Work out the finished part from the listing and answer in its coordinate system (mm). A direction names the side the tool comes from. Coordinates: 2 decimals unless noted, no trailing zeros. Order: outer loops, then holes, each group sorted by start corner. A loop starts at its lowest first (then second) coordinate and runs counter-clockwise, first axis right, second up. Notation, with made-up numbers: (68, -16) -> (104, -16) arc R16 cw to (104, -9) -> close; hole circle Ø10 at (80.5, 12.25). An arc over 180 degrees is marked (long way). Answer as CSV lines item,"result". Start each with the question number.
Item 1: Which of the six approach directions +Z, -Z, +X, -X, +Y, -Y give full straight-line access (tool end or side, diameter ignored) to faces 1 (the face through (1.972, -8.5, -5.156)), 2 (the face through (1.972, 6.461, -7.513)), 3 (the face through (1.972, 9.907, -0.825))?
Item 2: Section C-C (x = 4.75) is taken. Write down the section's boundary in (y, z).
Item 3: Each of these flat-tipped pins is pushed along its axis until it touches: pin 1 Ø4 at (x, y) = (19.5, 3) entering from +Z; pin 2 Ø6 at (x, z) = (8.5, -7.5) entering from +Y; pin 3 Ø2 at (x, y) = (20.5, 0) entering from -Z. Where does it stop, or does it pass through?
Item 4: Straight lines are drawn through the part: L1, parallel to X at y = -1, z = 6.25; L2, parallel to Y at x = 22.25, z = 0; L3, parallel to X at y = -9, z = 1.75. For each, find the intervals that lie inside material, in ascending order.
Item 5: Section A-A (z = 0) is taken. Write down the section's boundary in (x, y), then the cut area to 3 significant figures.
Item 6: Section D-D (y = -4.25) is taken. Write down the section's boundary in (x, z).
Item 7: For a pull along Z with two mould halves and no side action, classify faces 4 (the face through (1.972, 9.677, 2.277)), 5 (the face through (1.972, -0.811, 9.876)), 6 (the face through (0, 2, -2)) as pulls with the +Z half, pulls with the -Z half, needs draft (parallel to the pull), parting line crosses it, or undercut.
```python
from build123d import *

# Parameters (mm, degrees)
BASPROSKE_W             = 4
BASPROSKE_H             = 11
TOOTHCUT_DEPTH          = 17.062378404
TEETHCUTS_COUNT         = 20
TEETHCUTS_ANGLE         = 342
BORSKE_R                = 2.5
BORE_DEPTH              = 50.0000508
SKETCH1_R               = 8.5
BOSS_EXTRUDE1_DEPTH     = 4
SKETCH2_R               = 5
BOSS_EXTRUDE2_DEPTH     = 15
SKETCH3_R               = 8.5
BOSS_EXTRUDE3_DEPTH     = 5
SKETCH4_R               = 2.65
CUT_EXTRUDE1_DEPTH      = 32.964164392
CUT_EXTRUDE1_DEPTH_BACK = 32.964164392


with BuildPart() as part:
    # BasProSke → Base-Revolve (revolve)
    with BuildSketch(Plane(origin=(0, 0, 0), x_dir=(1, 0, 0), z_dir=(0, 1, 0)), mode=Mode.PRIVATE) as base_revolve_sk:
        with Locations((2, 5.5)):
            Rectangle(BASPROSKE_W, BASPROSKE_H)
    revolve(base_revolve_sk.sketch.rotate(Axis((-10, 0, 0), (1, 0, 0)), 180), axis=Axis((-10, 0, 0), (1, 0, 0)))

    # TooCutSke → ToothCut (cut, through all)
    with BuildSketch(Plane(origin=(0, 0, 0), x_dir=(0, 0, -1), z_dir=(1, 0, 0))):
        with BuildLine():
            ThreePointArc((0.499924007, 8.734705318), (0, 8.749), (-0.499924007, 8.734705318))
            ThreePointArc((-0.499924007, 8.734705318), (-0.824302243, 9.905497836), (-1.485192705, 10.924909509))
            ThreePointArc((-1.485192705, 10.924909509), (0, 11.0254), (1.485192705, 10.924909509))
            ThreePointArc((1.485192705, 10.924909509), (0.824302243, 9.905497836), (0.499924007, 8.734705318))
        make_face()
    toothcut = extrude(amount=TOOTHCUT_DEPTH, mode=Mode.SUBTRACT)

    # TeethCuts: ToothCut ×20 about axis
    teethcuts_axis = Axis((-10, 0, 0), (1, 0, 0))
    for i in range(1, TEETHCUTS_COUNT):
        add(toothcut.rotate(teethcuts_axis, i * TEETHCUTS_ANGLE / (TEETHCUTS_COUNT - 1)), mode=Mode.SUBTRACT)

    # BorSke → Bore (cut, symmetric)
    with BuildSketch(Plane(origin=(0, 0, 0), x_dir=(0, 0, -1), z_dir=(1, 0, 0))):
        with Locations(Location((0, 0, 0), (0, 0, 180))):
            Circle(BORSKE_R)
    extrude(amount=BORE_DEPTH, both=True, mode=Mode.SUBTRACT)

    # Sketch1 → Boss-Extrude1 (add)
    with BuildSketch(Plane(origin=(4, 0, 0), x_dir=(0, 0, -1), z_dir=(1, 0, 0))):
        with Locations(Location((0, 0, 0), (0, 0, 180))):
            Circle(SKETCH1_R)
    extrude(amount=BOSS_EXTRUDE1_DEPTH)

    # Sketch2 → Boss-Extrude2 (add)
    with BuildSketch(Plane(origin=(8, 0, 0), x_dir=(0, 0, -1), z_dir=(1, 0, 0))):
        Circle(SKETCH2_R)
    extrude(amount=BOSS_EXTRUDE2_DEPTH)

    # Sketch3 → Boss-Extrude3 (add)
    with BuildSketch(Plane(origin=(23, 0, 0), x_dir=(0, 0, -1), z_dir=(1, 0, 0))):
        with Locations(Location((0, 0, 0), (0, 0, 180))):
            Circle(SKETCH3_R)
    extrude(amount=BOSS_EXTRUDE3_DEPTH)

    # Sketch4 → Cut-Extrude1 (cut, two sides)
    with BuildSketch(Plane(origin=(28, 0, 0), x_dir=(0, 0, -1), z_dir=(1, 0, 0))) as cut_extrude1_sk:
        with Locations(Location((0, 0, 0), (0, 0, 180))):
            Circle(SKETCH4_R)
    extrude(amount=CUT_EXTRUDE1_DEPTH, mode=Mode.SUBTRACT)
    extrude(cut_extrude1_sk.sketch, amount=-CUT_EXTRUDE1_DEPTH_BACK, mode=Mode.SUBTRACT)


solid = part.part
```
Checked values:
1,face 1,"+X, -X"
1,face 2,"-Z, +X, -X"
1,face 3,"+X, -X, +Y"
2,outline,"circle Ø17 at (0, 0); hole circle Ø5.3 at (0, 0)"
3,pin 1,"stops at z = 4.9"
3,pin 2,"stops at y = 7.18"
3,pin 3,"stops at z = -5"
4,L1,"x = 0 to 8, 23 to 28"
4,L2,"y = -5 to -2.65, 2.65 to 5"
4,L3,"x = 0 to 4"
5,outline,"(0, -8.75) -> (4, -8.75) -> (4, -8.5) -> (8, -8.5) -> (8, -5) -> (23, -5) -> (23, -8.5) -> (28, -8.5) -> (28, -2.65) -> (0, -2.65) -> close; (0, 2.65) -> (28, 2.65) -> (28, 8.5) -> (23, 8.5) -> (23, 5) -> (8, 5) -> (8, 8.5) -> (4, 8.5) -> (4, 8.75) -> (0, 8.75) -> close"
5,area,"225 mm^2"
6,outline,"(0, -9.55) -> (4, -9.55) -> (4, -7.36) -> (8, -7.36) -> (8, -2.63) -> (23, -2.63) -> (23, -7.36) -> (28, -7.36) -> (28, 7.36) -> (23, 7.36) -> (23, 2.63) -> (8, 2.63) -> (8, 7.36) -> (4, 7.36) -> (4, 9.55) -> (0, 9.55) -> close"
7,face 4,"undercut"
7,face 5,"pulls with the +Z half"
7,face 6,"needs draft"
